from build123d import *

# Parameters (mm, degrees)
SKETCH1_W              = 66.5
SKETCH1_H              = 121.9
BOX_DEPTH              = 34.8
SKETCH4_W              = 62
SKETCH4_H              = 117.4
HOLLOW_DEPTH           = 32.55
SIDE_WALL_DRAFT_SIZE   = 34.8
SIDE_WALL_DRAFT_SIZE_2 = 1.1
CORNER_ROUNDING_R      = 4
SKETCH2_R              = 3.75
SKETCH2_R_2            = 4
SKETCH2_R_3            = 6
SKETCH2_R_4            = 3.175
TOP_SIDE_CUT_DEPTH     = 22.5
SKETCH6_R              = 5
INPUT_JACK_DEPTH       = 10
SKETCH7_R              = 5
OUTPUT_JACK_DEPTH      = 10


with BuildPart() as part:
    # Sketch1 → Box (new body)
    with BuildSketch(Plane(origin=(0, 0, 0), x_dir=(1, 0, 0), z_dir=(0, 1, 0))):
        Rectangle(SKETCH1_W, SKETCH1_H)
    extrude(amount=-BOX_DEPTH)

    # Sketch4 → Hollow (cut)
    with BuildSketch(Plane.XZ.offset(34.8)):
        Rectangle(SKETCH4_W, SKETCH4_H)
    extrude(amount=-HOLLOW_DEPTH, mode=Mode.SUBTRACT)

    # Side wall draft
    # the kernel refuses this chamfer: 34.8, 1.1 mm, written as the material it adds along each edge
    with BuildSketch(Plane(origin=(-31, -2.25, 58.7), x_dir=(-0.001215153825981483, -0.999999261700317, 0), z_dir=(0, 0, -1))) as side_wall_draft_piece_1_section:
        Polygon((SIDE_WALL_DRAFT_SIZE * 0.9999992617, -SIDE_WALL_DRAFT_SIZE * 0.00121515382598), (-SIDE_WALL_DRAFT_SIZE_2 * 0.00121515382598, -SIDE_WALL_DRAFT_SIZE_2 * 0.9999992617), (0, 0), align=None)
    side_wall_draft_piece_1 = extrude(amount=117.4, mode=Mode.PRIVATE)
    side_wall_draft_piece_1 = split(side_wall_draft_piece_1, bisect_by=Plane(origin=(-30.631893643, -34.8, 0), z_dir=(0, 1, 0)), keep=Keep.TOP, mode=Mode.PRIVATE)
    add(side_wall_draft_piece_1)
    with BuildSketch(Plane(origin=(31, -2.25, 58.7), x_dir=(0, -0.999999261700317, 0.0012151538259815812), z_dir=(-1, 0, 0))) as side_wall_draft_piece_2_section:
        Polygon((SIDE_WALL_DRAFT_SIZE * 0.9999992617, -SIDE_WALL_DRAFT_SIZE * 0.00121515382598), (-SIDE_WALL_DRAFT_SIZE_2 * 0.00121515382598, -SIDE_WALL_DRAFT_SIZE_2 * 0.9999992617), (0, 0), align=None)
    side_wall_draft_piece_2 = extrude(amount=62, mode=Mode.PRIVATE)
    side_wall_draft_piece_2 = split(side_wall_draft_piece_2, bisect_by=Plane(origin=(0, -34.8, 58.331893643), z_dir=(0, 1, 0)), keep=Keep.TOP, mode=Mode.PRIVATE)
    add(side_wall_draft_piece_2)
    with BuildSketch(Plane(origin=(31, -2.25, -58.7), x_dir=(0.001215153825981483, -0.999999261700317, 0), z_dir=(0, 0, 1))) as side_wall_draft_piece_3_section:
        Polygon((SIDE_WALL_DRAFT_SIZE * 0.9999992617, -SIDE_WALL_DRAFT_SIZE * 0.00121515382598), (-SIDE_WALL_DRAFT_SIZE_2 * 0.00121515382598, -SIDE_WALL_DRAFT_SIZE_2 * 0.9999992617), (0, 0), align=None)
    side_wall_draft_piece_3 = extrude(amount=117.4, mode=Mode.PRIVATE)
    side_wall_draft_piece_3 = split(side_wall_draft_piece_3, bisect_by=Plane(origin=(30.631893643, -34.8, 0), z_dir=(0, 1, 0)), keep=Keep.TOP, mode=Mode.PRIVATE)
    add(side_wall_draft_piece_3)
    with BuildSketch(Plane(origin=(-31, -2.25, -58.7), x_dir=(0, -0.999999261700317, -0.0012151538259815812), z_dir=(1, 0, 0))) as side_wall_draft_piece_4_section:
        Polygon((SIDE_WALL_DRAFT_SIZE * 0.9999992617, -SIDE_WALL_DRAFT_SIZE * 0.00121515382598), (-SIDE_WALL_DRAFT_SIZE_2 * 0.00121515382598, -SIDE_WALL_DRAFT_SIZE_2 * 0.9999992617), (0, 0), align=None)
    side_wall_draft_piece_4 = extrude(amount=62, mode=Mode.PRIVATE)
    side_wall_draft_piece_4 = split(side_wall_draft_piece_4, bisect_by=Plane(origin=(0, -34.8, -58.331893643), z_dir=(0, 1, 0)), keep=Keep.TOP, mode=Mode.PRIVATE)
    add(side_wall_draft_piece_4)
    # the kernel refuses this chamfer: 34.8, 1.1 mm, written as the material it takes off along each edge
    with BuildSketch(Plane(origin=(-123.728329596, 0, 60.95), x_dir=(0, -0.999999261700317, 0.0012151538259815812), z_dir=(1, 0, 0))) as side_wall_draft_2_piece_1:
        Polygon((SIDE_WALL_DRAFT_SIZE * 0.9999992617, SIDE_WALL_DRAFT_SIZE * 0.00121515382598), (-SIDE_WALL_DRAFT_SIZE_2 * 0.00121515382598, SIDE_WALL_DRAFT_SIZE_2 * 0.9999992617), (0, 0), align=None)
    extrude(amount=247.456659192, mode=Mode.SUBTRACT)
    with BuildSketch(Plane(origin=(-33.25, 0, -151.428329596), x_dir=(-0.0012151538259815812, -0.999999261700317, 0), z_dir=(0, 0, 1)), Plane(origin=(33.25, 0, 151.428329596), x_dir=(0.0012151538259815812, -0.999999261700317, 0), z_dir=(0, 0, -1))) as side_wall_draft_2_piece_2:
        Polygon((SIDE_WALL_DRAFT_SIZE * 0.9999992617, SIDE_WALL_DRAFT_SIZE * 0.00121515382598), (-SIDE_WALL_DRAFT_SIZE_2 * 0.00121515382598, SIDE_WALL_DRAFT_SIZE_2 * 0.9999992617), (0, 0), align=None)
    extrude(amount=302.856659192, mode=Mode.SUBTRACT)
    with BuildSketch(Plane(origin=(123.728329596, 0, -60.95), x_dir=(0, 0.7724211149227607, 0.6351107157192984), z_dir=(-1, 0, 0))) as side_wall_draft_2_piece_3:
        Polygon((SIDE_WALL_DRAFT_SIZE_2 * 0.635110715719, -SIDE_WALL_DRAFT_SIZE_2 * 0.772421114923), (-SIDE_WALL_DRAFT_SIZE * 0.772421114923, -SIDE_WALL_DRAFT_SIZE * 0.635110715719), (0, 0), align=None)
    extrude(amount=247.456659192, mode=Mode.SUBTRACT)

    # Corner rounding
    corner_rounding_edges = [part.edges().sort_by_distance(p)[0] for p in [
        (0, -2.25, -57.6),
        (29.9, -2.25, 0),
        (0, -2.25, 57.6),
        (-29.9, -2.25, 0),
        (32.15, 0, 0),
        (0, 0, -59.85),
        (-32.15, 0, 0),
        (0, 0, 59.85),
        (30.414439655, -18.525, 58.114439655),
        (30.414439655, -18.525, -58.114439655),
        (-30.414439655, -18.525, 58.114439655),
        (-30.414439655, -18.525, -58.114439655),
        (-32.7, -17.4, -60.4),
        (32.7, -17.4, -60.4),
        (-32.7, -17.4, 60.4),
        (32.7, -17.4, 60.4),
    ]]
    fillet(corner_rounding_edges, radius=CORNER_ROUNDING_R)

    # Sketch2 → Top side cut (cut)
    with BuildSketch(Plane(origin=(0, 0, 0), x_dir=(1, 0, 0), z_dir=(0, 1, 0))):
        with Locations(Location((-18, 40, 0), (0, 0, 270))):
            Circle(SKETCH2_R)
        with Locations(Location((0, -13.75, 0), (0, 0, 270))):
            Circle(SKETCH2_R_2)
        with Locations(Location((0, -31.5, 0), (0, 0, 270))):
            Circle(SKETCH2_R_3)
        with Locations(Location((-20, 12.5, 0), (0, 0, 270))):
            Circle(SKETCH2_R_4)
        with Locations(Location((18, 40, 0), (0, 0, 270))):
            Circle(SKETCH2_R)
        with Locations(Location((0, 10, 0), (0, 0, 270))):
            Circle(SKETCH2_R)
    extrude(amount=-TOP_SIDE_CUT_DEPTH, mode=Mode.SUBTRACT)

    # Sketch6 → Input Jack (cut)
    with BuildSketch(Plane(origin=(32.117909672, 1.015221283, 0), x_dir=(0, 0, -1), z_dir=(0.9995008034277885, 0.03159341620030004, 0))):
        with Locations(Location((-5, -18.415728331, 0), (0, 0, 90))):
            Circle(SKETCH6_R)
    extrude(amount=-INPUT_JACK_DEPTH, mode=Mode.SUBTRACT)

    # Sketch7 → Output Jack (cut)
    with BuildSketch(Plane(origin=(-32.117909672, 1.015221283, 0), x_dir=(0, 0, 1), z_dir=(-0.9995008034277885, 0.03159341620030004, 0))):
        with Locations(Location((5, -18.293286119, 0), (0, 0, 270))):
            Circle(SKETCH7_R)
    extrude(amount=-OUTPUT_JACK_DEPTH, mode=Mode.SUBTRACT)


solid = part.part
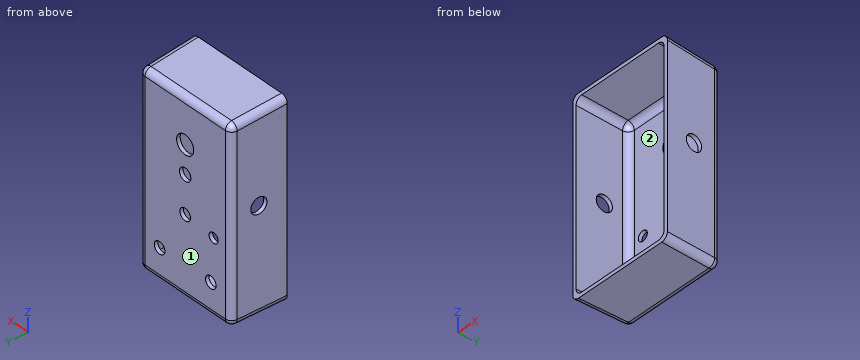
Source: CAD feature listing. Evaluate the final solid. Frame: model axes, mm. Face numbers are marked on the shaded views. Round coordinates to 2 decimals unless told otherwise and drop trailing zeros. Loops run counter-clockwise (first coordinate to the right, second up) from the corner with the lowest first, then second, coordinate; pieces in that order, holes last. Notation, with made-up numbers: M -18.75,-32 L 31.25,-32 A22 cw 31.25,-14 Z; hole C 40,-37 d3. An arc over 180 degrees is marked long. Answer as CSV lines item,"result".
Q1. Cut plane A-A (z = 31.5). Return the cut outline in (x, y).
Verdict:
outline,"M -33.25,-34.8 L -30.93,-34.8 L -30.02,-6.12 A4 cw -26.02,-2.25 L -6,-2.25 L -6,0 L -28.27,0 A4 ccw -32.27,-3.87 Z; M 6,-2.25 L 26.02,-2.25 A4 cw 30.02,-6.12 L 30.93,-34.8 L 33.25,-34.8 L 32.27,-3.87 A4 ccw 28.27,0 L 6,0 Z"
Q2. Pull-direction query (X, two-part tool) for the marked faces 1 and 2; classes: +X half, -X half, draft (parallel to the pull), parting line (faces both ways), or undercut.
Verdict:
face 1,"draft"
face 2,"undercut"
Q3. Line query: line 1 along X through (y, z) = (-1, -40); line 2 along Y through (x, z) = (-6.5, 17); line 3 along X through (y, z) = (-11, -3). Output: solid intervals per line, ascending.
Verdict:
line 1,"x = -30.92 to -21.75, -14.25 to 14.25, 21.75 to 30.92"
line 2,"y = -2.25 to 0"
line 3,"x = -32.5 to -30.18, 30.18 to 32.5"
Q4. Cut plane B-B (z = -40). Return the cut outline in (x, y).
Verdict:
outline,"M -33.25,-34.8 L -30.93,-34.8 L -30.02,-6.12 A4 cw -26.02,-2.25 L -21.75,-2.25 L -21.75,0 L -28.27,0 A4 ccw -32.27,-3.87 Z; M -14.25,-2.25 L 14.25,-2.25 L 14.25,0 L -14.25,0 Z; M 21.75,-2.25 L 26.02,-2.25 A4 cw 30.02,-6.12 L 30.93,-34.8 L 33.25,-34.8 L 32.27,-3.87 A4 ccw 28.27,0 L 21.75,0 Z"
Q5. Cut plane C-C (x = 0). Return the cut outline in (y, z).
Verdict:
outline,"M -34.8,-60.95 L -3.87,-59.97 A4 ccw 0,-55.97 L 0,-13.75 L -2.25,-13.75 L -2.25,-53.72 A4 cw -6.12,-57.72 L -34.8,-58.63 Z; M -34.8,58.63 L -6.12,57.72 A4 cw -2.25,53.72 L -2.25,37.5 L 0,37.5 L 0,55.97 A4 ccw -3.87,59.97 L -34.8,60.95 Z; M -2.25,-6.25 L 0,-6.25 L 0,9.75 L -2.25,9.75 Z; M -2.25,17.75 L 0,17.75 L 0,25.5 L -2.25,25.5 Z"
Q6. Cut plane D-D (x = -18). Return the cut outline in (y, z).
Verdict:
outline,"M -34.8,-60.95 L -3.87,-59.97 A4 ccw 0,-55.97 L 0,-43.75 L -2.25,-43.75 L -2.25,-53.72 A4 cw -6.12,-57.72 L -34.8,-58.63 Z; M -34.8,58.63 L -6.12,57.72 A4 cw -2.25,53.72 L -2.25,-10.03 L 0,-10.03 L 0,55.97 A4 ccw -3.87,59.97 L -34.8,60.95 Z; M -2.25,-36.25 L 0,-36.25 L 0,-14.97 L -2.25,-14.97 Z"
Q7. Contact query for flat-ended pins moving along their axis: pin 1 (3 mm diameter, centred on x = 26, y = -14.5, fed in from +Z); pin 2 (6 mm diameter, centred on y = -17, z = -27.5, fed in from -X); pin 3 (12 mm diameter, centred on x = -21, y = -25, fed in from +Z); pin 4 (5 mm diameter, centred on x = -20, z = -12.5, fed in from -Y). Output: stop coordinate, or through.
Verdict:
pin 1,"stops at z = 60.36"
pin 2,"stops at x = -32.78"
pin 3,"stops at z = 60.83"
pin 4,"passes through"
